Could you check a few things on this model? Use its own coordinates, in mm. Give positions to 0.01 mm unless a question says otherwise; leave off trailing zeros. Order: outer loops, then holes, each group sorted by start corner. A loop starts at its lowest first (then second) coordinate and runs counter-clockwise, first axis right, second up. Notation, with made-up numbers: (64, 81) - (103, 81) arc R16 cw to (103, 102) - close; hole circle Ø5 at (80.5, 41.25). An arc over 180 degrees is marked (long way). Put each result on its own line as item: value.
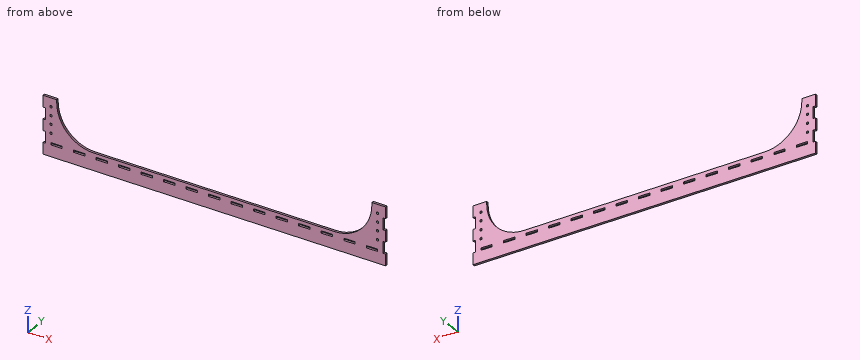
from build123d import *

# Parameters (mm, degrees)
SKETCH1_R           = 2.125
SKETCH1_W           = 19.725
SKETCH1_H           = 4
BOSS_EXTRUDE1_DEPTH = 4


with BuildPart() as part:
    # Sketch1 → Boss-Extrude1 (new body)
    with BuildSketch(Plane(origin=(0, 0, 0), x_dir=(1, 0, 0), z_dir=(0, 1, 0))):
        with BuildLine():
            Line((299.8, 24), (299.8, 4))
            Line((299.8, 4), (295.8, 4))
            Line((295.8, 4), (295.8, -16))
            Line((295.8, -16), (299.8, -16))
            Line((299.8, -16), (299.8, -36))
            Line((299.8, -36), (295.8, -36))
            Line((295.8, -36), (295.8, -56))
            Line((295.8, -56), (299.8, -56))
            Line((299.8, -56), (299.8, -76))
            Line((299.8, -76), (275.8, -76))
            Line((275.8, -76), (275.8, -71))
            ThreePointArc((275.8, -71), (256.761940777, -25.038059223), (210.8, -6))
            Line((210.8, -6), (-210.8, -6))
            ThreePointArc((-210.8, -6), (-256.761940777, -25.038059223), (-275.8, -71))
            Line((-275.8, -71), (-275.8, -76))
            Line((-275.8, -76), (-299.8, -76))
            Line((-299.8, -76), (-299.8, -56))
            Line((-299.8, -56), (-295.8, -56))
            Line((-295.8, -56), (-295.8, -36))
            Line((-295.8, -36), (-299.8, -36))
            Line((-299.8, -36), (-299.8, -16))
            Line((-299.8, -16), (-295.8, -16))
            Line((-295.8, -16), (-295.8, 4))
            Line((-295.8, 4), (-299.8, 4))
            Line((-299.8, 4), (-299.8, 24))
            Line((-299.8, 24), (299.8, 24))
        make_face()
        with Locations((285.8, -61)):
            Circle(SKETCH1_R, mode=Mode.SUBTRACT)
        with Locations((285.8, -46)):
            Circle(SKETCH1_R, mode=Mode.SUBTRACT)
        with Locations((-285.8, -46)):
            Circle(SKETCH1_R, mode=Mode.SUBTRACT)
        with Locations((-285.8, -61)):
            Circle(SKETCH1_R, mode=Mode.SUBTRACT)
        with Locations((285.8, -16)):
            Circle(SKETCH1_R, mode=Mode.SUBTRACT)
        with Locations((285.8, -31)):
            Circle(SKETCH1_R, mode=Mode.SUBTRACT)
        with Locations((-285.8, -31)):
            Circle(SKETCH1_R, mode=Mode.SUBTRACT)
        with Locations((-285.8, -16)):
            Circle(SKETCH1_R, mode=Mode.SUBTRACT)
        with Locations((0, 2)):
            Rectangle(SKETCH1_W, SKETCH1_H, mode=Mode.SUBTRACT)
        with Locations((39.45, 2)):
            Rectangle(SKETCH1_W, SKETCH1_H, mode=Mode.SUBTRACT)
        with Locations((78.87, 2)):
            Rectangle(SKETCH1_W, SKETCH1_H, mode=Mode.SUBTRACT)
        with Locations((118.29, 2)):
            Rectangle(SKETCH1_W, SKETCH1_H, mode=Mode.SUBTRACT)
        with Locations((157.71, 2)):
            Rectangle(SKETCH1_W, SKETCH1_H, mode=Mode.SUBTRACT)
        with Locations((197.13, 2)):
            Rectangle(SKETCH1_W, SKETCH1_H, mode=Mode.SUBTRACT)
        with Locations((236.55, 2)):
            Rectangle(SKETCH1_W, SKETCH1_H, mode=Mode.SUBTRACT)
        with Locations((275.97, 2)):
            Rectangle(SKETCH1_W, SKETCH1_H, mode=Mode.SUBTRACT)
        with Locations((-275.97, 2)):
            Rectangle(SKETCH1_W, SKETCH1_H, mode=Mode.SUBTRACT)
        with Locations((-236.55, 2)):
            Rectangle(SKETCH1_W, SKETCH1_H, mode=Mode.SUBTRACT)
        with Locations((-197.13, 2)):
            Rectangle(SKETCH1_W, SKETCH1_H, mode=Mode.SUBTRACT)
        with Locations((-157.71, 2)):
            Rectangle(SKETCH1_W, SKETCH1_H, mode=Mode.SUBTRACT)
        with Locations((-118.29, 2)):
            Rectangle(SKETCH1_W, SKETCH1_H, mode=Mode.SUBTRACT)
        with Locations((-78.87, 2)):
            Rectangle(SKETCH1_W, SKETCH1_H, mode=Mode.SUBTRACT)
        with Locations((-39.45, 2)):
            Rectangle(SKETCH1_W, SKETCH1_H, mode=Mode.SUBTRACT)
    extrude(amount=BOSS_EXTRUDE1_DEPTH)


solid = part.part
1) Suppose I cut it at B-B, the plane x = -135.5. List the corners of the cut face in (y, z) for me, and give its area (3 significant figures).
Filled in:
outline: (0, -24) - (4, -24) - (4, 6) - (0, 6) - close
area: 120 mm^2
2) I'm going to push flat-ended pins straight in: pin 1 (2 mm diameter, centred on y = 2.5, z = -1, fed in from +X); pin 2 (2 mm diameter, centred on y = 3, z = -2.5, fed in from -X). Where does each tip first touch, or does it pass through?
Filled in:
pin 1: stops at x = 295.8
pin 2: stops at x = -295.8
3) Suppose I cut it at A-A, the plane y = 1.4. State how many separate pieces and enclosed holes the cut face has, and give its area (3 significant figures).
Filled in:
separate pieces: 1
enclosed holes: 23
area: 21,500 mm^2
4) If I drill on line 1 (Z direction, x = 285.8, y = 1.75) (3 decimals); line 2 (X direction, y = 0.5, z = 67.5); line 3 (X direction, y = 2.1, z = 46) (3 decimals), over which ranges is the centre line in solid material (lowest first)? Write a range as [from, to].
Filled in:
line 1: z = [-24, -4], [0, 13.875], [18.125, 28.875], [33.125, 43.875], [48.125, 58.875], [63.125, 76]
line 2: x = [-299.8, -275.71], [275.71, 299.8]
line 3: x = [-295.8, -287.925], [-283.675, -270.8], [270.8, 283.675], [287.925, 295.8]
